Job drawing, mm, ordinate dimensions from the low corner. One solid piece. Round coordinates to 2 decimals unless told otherwise and drop trailing zeros. Loops run counter-clockwise (first coordinate to the right, second up) from the corner with the lowest first, then second, coordinate; pieces in that order, holes last.
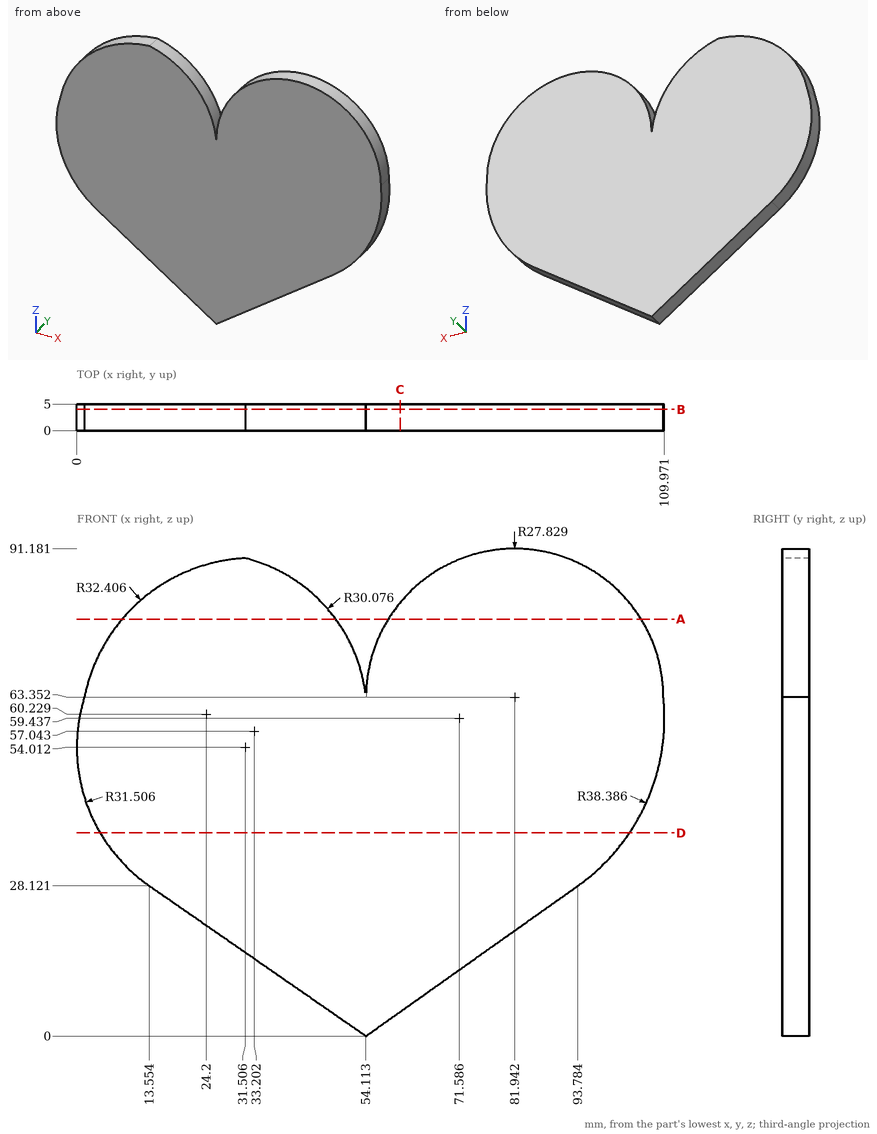
(1) Slice it at B-B on y = 4. List the corners of the cut face in (x, z) (1 decimal), plus the area to 3 significant figures.
Responses:
outline: (1.4, 63.4) arc R31.5 ccw to (13.6, 28.1) - (54.1, 0) - (93.8, 28.1) arc R38.4 ccw to (109.8, 63.4) arc R27.8 ccw to (54.1, 63.4) arc R30.1 ccw to (31.5, 89.4) arc R32.4 ccw to start
area: 6,960 mm2
(2) Slice it at D-D on z = 38. List the corners of the cut face in (x, y).
Responses:
outline: (4.37, 0) - (103.43, 0) - (103.43, 5) - (4.37, 5) - close
(3) Pin check, flat tips, straight feed: P1, Ø2, axis at y = 1.5, z = 28.5, coming from the -X side (1 decimal); P2, Ø6, axis at x = 32, z = 26, coming from the -Y side; P3, Ø1, axis at y = 1.5, z = 73, coming from the -X side. Stop position of each tip, or through.
Responses:
P1: stops at x = 11.7
P2: stops at y = 0
P3: stops at x = 4.72
(4) Slice it at C-C on x = 60.5. List the corners of the cut face in (y, z).
Responses:
outline: (0, 4.53) - (5, 4.53) - (5, 81.09) - (0, 81.09) - close
(5) Slice it at A-A on z = 78. List the corners of the cut face in (x, y) (1 decimal).
Responses:
outline: (8.5, 0) - (48.5, 0) - (48.5, 5) - (8.5, 5) - close; (58.3, 0) - (105.6, 0) - (105.6, 5) - (58.3, 5) - close
(6) Probe line 1 (X direction, y = 3.8, z = 69); line 2 (X direction, y = 3.15, z = 66.5) (1 decimal); line 3 (Z direction, x = 61.5, y = 4) (1 decimal). List the from-to ranges inside material, lowest first.
Responses:
line 1: x = 3.08 to 52.97, 54.69 to 109.19
line 2: x = 2.2 to 53.6, 54.3 to 109.6
line 3: z = 5.2 to 82.2
